Design review of the part built by this model. Coordinates are the model's own, in mm. A direction names the side the tool comes from. Coordinates: 2 decimals unless noted, no trailing zeros. Write each loop counter-clockwise with the first axis right and the second up, starting at its lowest first coordinate (ties: lowest second). Pieces come first, ordered by that corner, then holes.
```python
from build123d import *

# Parameters (mm, degrees)
SKETCH1_W               = 51.4
SKETCH1_H               = 4.5
BOSS_EXTRUDE1_DEPTH     = 10
CUT_EXTRUDE1_DEPTH      = 47.230988755
CUT_EXTRUDE1_DEPTH_BACK = 47.230988755
SKETCH2_R               = 2.15
SKETCH3_W               = 14
SKETCH3_H               = 3
BOSS_EXTRUDE2_DEPTH     = 20
CUT_EXTRUDE2_DEPTH      = 20
FILLET1_R               = 1


with BuildPart() as part:
    # Sketch1 → Boss-Extrude1 (new body)
    with BuildSketch(Plane.XY):
        with Locations((19.211627907, 1.395348837)):
            Rectangle(SKETCH1_W, SKETCH1_H)
    extrude(amount=BOSS_EXTRUDE1_DEPTH)

    # Sketch2 → Cut-Extrude1 (cut, two sides: drawn at the far end of the back side and taken through both)
    with BuildSketch(Plane(origin=(0, 3.645348837, 0), x_dir=(1, 0, 0), z_dir=(0, 1, 0)).offset(-CUT_EXTRUDE1_DEPTH_BACK)):
        with Locations(Location((-3.488372093, -5, 0), (0, 0, 270))):
            Circle(SKETCH2_R)
        with Locations(Location((41.911627907, -5, 0), (0, 0, 270))):
            Circle(SKETCH2_R)
    extrude(amount=CUT_EXTRUDE1_DEPTH + CUT_EXTRUDE1_DEPTH_BACK, mode=Mode.SUBTRACT)

    # Sketch3 → Boss-Extrude2 (add)
    with BuildSketch(Plane(origin=(0, 3.645348837, 0), x_dir=(1, 0, 0), z_dir=(0, 1, 0))):
        with Locations((19.211627907, -1.5)):
            Rectangle(SKETCH3_W, SKETCH3_H)
    extrude(amount=BOSS_EXTRUDE2_DEPTH)

    # Sketch4 → Cut-Extrude2 (cut)
    with BuildSketch(Plane.XY.offset(3)):
        with BuildLine():
            Line((17.211627907, 21.145348837), (21.211627907, 21.145348837))
            ThreePointArc((21.211627907, 21.145348837), (23.211627907, 19.145348837), (21.211627907, 17.145348837))
            Line((21.211627907, 17.145348837), (17.211627907, 17.145348837))
            ThreePointArc((17.211627907, 17.145348837), (15.211627907, 19.145348837), (17.211627907, 21.145348837))
        make_face()
    extrude(amount=-CUT_EXTRUDE2_DEPTH, mode=Mode.SUBTRACT)

    # Fillet1
    fillet1_edges = [part.edges().sort_by_distance(p)[0] for p in [
        (19.211627907, 3.645348837, 10),
        (2.861627907, 3.645348837, 0),
        (12.211627907, 3.645348837, 1.5),
        (12.211627907, 13.645348837, 0),
        (19.211627907, 3.645348837, 3),
        (12.211627907, 13.645348837, 3),
        (26.211627907, 3.645348837, 1.5),
        (26.211627907, 13.645348837, 3),
        (26.211627907, 13.645348837, 0),
        (12.211627907, 23.645348837, 1.5),
        (19.211627907, 23.645348837, 3),
        (26.211627907, 23.645348837, 1.5),
        (35.561627907, 3.645348837, 0),
    ]]
    fillet(fillet1_edges, radius=FILLET1_R)


solid = part.part
```
(1) Consider section B-B (y = 12.25). Give the boundary of the cut face in (x, z), plus the area to 3 significant figures.
(2) Mouldability with a two-part tool opening along Y and no side actions: class faces 5 (the flat face through (19, 23.645, 1)), 6 (the cylindrical face through (25.911, 14.278, 0.285)), 7 (the cylindrical face through (23.21, 19.19, 1.52)), 8 (the cylindrical face through (15.212, 19.101, 1.521)) as +Y half, -Y half, draft (parallel to the pull), parting line (faces both ways), or undercut.
(3) For faces 1 (the flat face through (12.212, 13.5, 1.5)), 2 (the cylindrical face through (12.5, 14.3, 0.3)), 3 (the flat face through (19, 3.645, 5)), 4 (the flat face through (26.212, 13.5, 1.5)), list the 3-axis set-ups (+Z, -Z, +X, -X, +Y, -Y) from which the entire face can be reached by the end or side of a thin tool; tool diameter is ignored.
(4) Consider section A-A (z = 5). Give the boundary of the cut face in (x, y), plus the area to 3 significant figures.
(5) Wall thickness on line 1 (X direction, y = 2.1, z = 5); line 2 (X direction, y = 1.5, z = 6.5); line 3 (Y direction, x = 15, z = 8): over which ranges is each line inside the solid? List them lowest first.
(6) Consider section C-C (x = 14). Give the boundary of the cut face in (y, z), plus the area to 3 significant figures.
(7) Insertion check: pin 1 Ø1.1 at (y, z) = (9.5, 1.5) entering from -X; pin 2 Ø5 at (x, z) = (32.5, 1.5) entering from +Y; pin 3 Ø1.1 at (y, z) = (10.5, 1.5) entering from +X. Each pin has a flat end and moves straight along its axis. Give the tip position at first contact, or say it passes through.
Results:
1. outline: (12.21, 1) arc R1 ccw to (13.21, 0) - (25.21, 0) arc R1 ccw to (26.21, 1) - (26.21, 2) arc R1 ccw to (25.21, 3) - (13.21, 3) arc R1 ccw to (12.21, 2) - close
1. area: 41.1 mm2
2. face 5: +Y half
2. face 6: draft
2. face 7: undercut
2. face 8: undercut
3. face 1: +Z, -Z, -X, +Y
3. face 2: -Z, -X, +Y
3. face 3: +Z, +Y
3. face 4: +Z, -Z, +X, +Y
4. outline: (-6.49, -0.85) - (-5.64, -0.85) - (-5.64, 3.65) - (-6.49, 3.65) - close; (-1.34, -0.85) - (39.76, -0.85) - (39.76, 3.65) - (-1.34, 3.65) - close; (44.06, -0.85) - (44.91, -0.85) - (44.91, 3.65) - (44.06, 3.65) - close
4. area: 193 mm2
5. line 1: x = -6.49 to -5.64, -1.34 to 39.76, 44.06 to 44.91
5. line 2: x = -6.49 to -5.03, -1.95 to 40.37, 43.45 to 44.91
5. line 3: y = -0.85 to 3.65
6. outline: (-0.85, 0) - (23.65, 0) - (23.65, 2) arc R1 ccw to (22.65, 3) - (4.65, 3) arc R1 cw to (3.65, 4) - (3.65, 9) arc R1 ccw to (2.65, 10) - (-0.85, 10) - close
6. area: 105 mm2
7. pin 1: stops at x = 12.21
7. pin 2: stops at y = 3.65
7. pin 3: stops at x = 26.21
